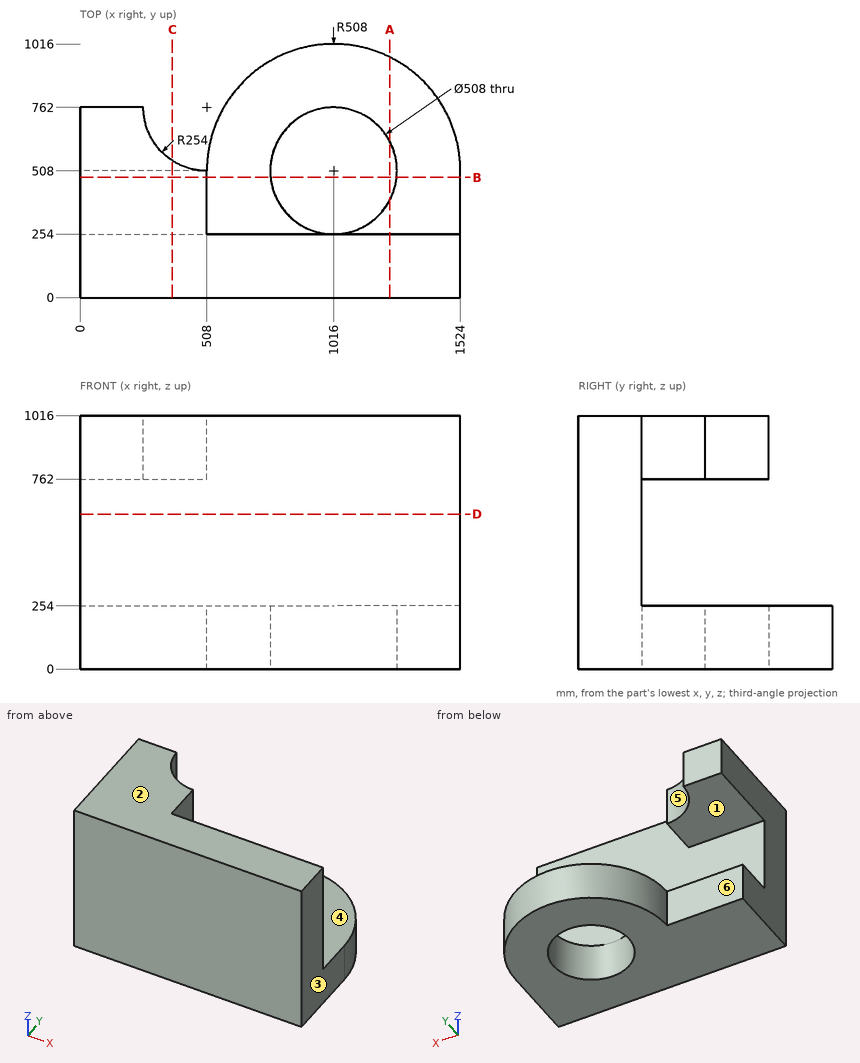
The figure shows three views and two pictorial views of one solid part (mm, origin at its lowest corner). Answer the questions. A direction names the side the tool comes from. Round coordinates to 2 decimals unless told otherwise and drop trailing zeros. Write each loop counter-clockwise with the first axis right and the second up, starting at its lowest first coordinate (ties: lowest second). Pieces come first, ordered by that corner, then holes. Notation, with made-up numbers: M 76,-15.5 L 93,-15.5 A20 ccw 93,-4.5 Z; hole C 9,-35.75 d5. An arc over 180 degrees is marked long. Write each question's results on one line, items separated by ' | '. Start each with the question number.
(1) For the marked faces 4, 5 and 6, determine the directions among +Z, -Z, +X, -X, +Y, -Y from which every point of the face is accessible in a straight line to the end or side of a thin tool.
(2) The part is cut by section A-A, the plane x = 1241. Write down the section's boundary in (y, z).
(3) The part is cut by section B-B, the plane y = 481.5. Write down the section's boundary in (x, z).
(4) The part is cut by section D-D, the plane z = 621.5. Write down the section's boundary in (x, y), and give its area (3 significant figures).
(5) Determine the mould class of the marked faces 1, 2 and 3 for opening direction Z: +Z half, -Z half, draft (parallel to the pull), parting line (faces both ways), or undercut.
(6) The part is cut by section C-C, the plane x = 370. Write down the section's boundary in (y, z).
(7) Each of these flat-tipped pins is pushed along its axis until it touches: P1, Ø5, axis at x = 747.5, z = 662, coming from the -Y side; P2, Ø5, axis at x = 1064, z = 501, coming from the +Y side; P3, Ø5, axis at y = 389, z = 859, coming from the +X side; P4, Ø8, axis at x = 650.5, z = 225, coming from the +Y side. Where does it stop, or does it pass through?
(8) Find the intervals of material crossed by line 1 (Y direction, x = 1016, z = 121); line 2 (Y direction, x = 323.5, z = 138); line 3 (Y direction, x = 468.5, z = 623), in increasing order.
Worked answers:
1) face 4: +X, -X, +Y | face 5: +Z, -Z, +X, +Y | face 6: -Z, -X, +Y
2) outline: M 0,0 L 390.14,0 L 390.14,254 L 254,254 L 254,1016 L 0,1016 Z; M 625.86,0 L 963.45,0 L 963.45,254 L 625.86,254 Z
3) outline: M 0,0 L 763.39,0 L 763.39,254 L 0,254 Z; M 0,762 L 508,762 L 508,1016 L 0,1016 Z; M 1268.61,0 L 1524,0 L 1524,254 L 1268.61,254 Z
4) outline: M 0,0 L 1524,0 L 1524,254 L 0,254 Z | area: 387,000 mm²
5) face 1: undercut | face 2: +Z half | face 3: draft
6) outline: M 0,0 L 508,0 L 508,254 L 254,254 L 254,762 L 548.76,762 L 548.76,1016 L 0,1016 Z
7) P1: stops at y = 0 | P2: stops at y = 254 | P3: stops at x = 508 | P4: stops at y = 864.91
8) line 1: y = 0 to 254, 762 to 1016 | line 2: y = 0 to 508 | line 3: y = 0 to 254
